Autodesk Inventor part; units mm, degrees
ref_plane "YZ Plane" through (0, 0, 0) normal (1, 0, 0) x (0, 1, 0)
ref_plane "XZ Plane" through (0, 0, 0) normal (0, 1, 0) x (-1, 0, 0)
ref_plane "XY Plane" through (0, 0, 0) normal (0, 0, 1) x (1, 0, 0)
sketch "Sketch1" plane through (0, 0, 0) normal (0, 0, 1) x (1, 0, 0)
  circle A0 centre (0, 0) radius 75 construction
  arc A1 (-78.5195, 32.5529) -> (0, 0) centre (-15.5934, 73.3611) ccw
  line L0 (-15.5934, 73.3611) -> (-78.5195, 32.5529) construction
  line L1 (-15.5934, 73.3611) -> (0, 0) construction
  line L2 (0, 0) -> (64.9519, 37.5) construction
  arc A2 (6.6958, 84.7359) -> (0, 0) centre (64.9519, 37.5) ccw
  line L3 (64.9519, 37.5) -> (6.6958, 84.7359) construction
  line L4 (64.9519, 37.5) -> (0, 0) construction
  line L5 (0, 0) -> (0, 75) construction
  circle A3 centre (0, 0) radius 85 construction
  arc A4 (6.6958, 84.7359) -> (-78.5195, 32.5529) centre (0, 0) ccw
  arc A5 (-74.153, 41.5492) -> (-78.5195, 32.5529) centre (-76.3362, 37.0511) ccw
  line L6 (-76.3362, 37.0511) -> (-78.5195, 32.5529) construction
  line L7 (-76.3362, 37.0511) -> (-74.153, 41.5492) construction
  point P0 (0, 0)
  dimension "d1" = 72
  dimension "d4" = 60
  dimension "d21" = 170
  dimension "d39" = 5
  dimension "d40" = 180
extrude "Extrusion1" add sketch "Sketch1" along normal blind 10
sketch "Sketch3" plane through (0, 0, 10) normal (0, 0, 1) x (1, 0, 0)
  circle A0 centre (0, 0) radius 80 construction
  circle A1 centre (64.9519, 37.5) radius 75
  circle A2 centre (64.9519, 37.5) radius 80 construction
  point P0 (0, 0)
  point P1 (-2.8573, 79.949)
  dimension "d25" = 160
  dimension "d26" = 160
hole "Hole2" at (-2.8573, 79.949, 10) direction (0, 0, -1) diameter 5 end through all
sketch "Sketch4" plane through (0, 0, 10) normal (0, 0, 1) x (1, 0, 0)
  circle A0 centre (-2.8573, 79.949) radius 2.5
  arc A1 (-78.5195, 32.5529) -> (0, 0) centre (-15.5934, 73.3611) ccw
  arc A2 (6.6958, 84.7359) -> (1.3808, 77.2959) centre (64.9519, 37.5) ccw
  arc A3 (6.6958, 84.7359) -> (-3.0359, 84.9458) centre (0, 0) ccw
  arc A4 (6.6958, 84.7359) -> (0, 0) centre (64.9519, 37.5) ccw
  arc A5 (6.6958, 84.7359) -> (-78.5195, 32.5529) centre (0, 0) ccw
  circle A6 centre (-2.8573, 79.949) radius 5
extrude "Extrusion2" cut sketch "Sketch4" against normal blind 10 contours A3 A2 A6
sketch "Sketch5" plane through (0, 0, 10) normal (0, 0, 1) x (1, 0, 0)
  arc A0 (1.3808, 77.2959) -> (-3.0359, 84.9458) centre (-2.8573, 79.949) ccw
  arc A1 (-3.0359, 84.9458) -> (-74.153, 41.5492) centre (0, 0) ccw
  arc A2 (-74.153, 41.5492) -> (-78.5195, 32.5529) centre (-76.3362, 37.0511) ccw
  arc A3 (-78.5195, 32.5529) -> (0, 0) centre (-15.5934, 73.3611) ccw
  arc A4 (1.3808, 77.2959) -> (0, 0) centre (64.9519, 37.5) ccw
  circle A5 centre (-2.8573, 79.949) radius 2.5
  point P0 (0, 0)
hole "Hole3" at (-76.3362, 37.0511, 10) direction (0, 0, -1) diameter 4.134 end through all
sketch "Sketch7" plane through (0, 0, 0) normal (0, 0, -1) x (-1, 0, 0)
  circle A0 centre (76.3362, 37.0511) radius 2.067
  arc A1 (3.0359, 84.9458) -> (-1.3808, 77.2959) centre (2.8573, 79.949) ccw
  arc A2 (0, 0) -> (-1.3808, 77.2959) centre (-64.9519, 37.5) ccw
  arc A3 (0, 0) -> (78.5195, 32.5529) centre (15.5934, 73.3611) ccw
  arc A4 (78.5195, 32.5529) -> (74.153, 41.5492) centre (76.3362, 37.0511) ccw
  arc A5 (74.153, 41.5492) -> (3.0359, 84.9458) centre (0, 0) ccw
  circle A6 centre (2.8573, 79.949) radius 2.5
  arc A7 (71.5064, 35.8724) -> (12.5647, 79.0071) centre (0, 0) ccw
  arc A8 (14.8454, 3.3651) -> (70.9945, 30.5742) centre (15.5934, 73.3611) ccw
  arc A9 (10.2017, 10.0786) -> (7.2658, 71.9181) centre (-64.9519, 37.5) ccw
  arc A10 (10.2017, 10.0786) -> (14.8454, 3.3651) centre (14.8988, 8.3648) ccw
  arc A11 (12.5647, 79.0071) -> (7.2658, 71.9181) centre (11.7794, 74.0692) ccw
  arc A12 (70.9945, 30.5742) -> (71.5064, 35.8724) centre (67.0373, 33.6304) ccw
  point P0 (0, 0)
  dimension "d51" = 5
  dimension "d55" = 5
extrude "Extrusion4" cut sketch "Sketch7" against normal blind 2 contours A12 A8 A10 A9 A11 A7
properties part number "blad"
Read the model definition and answer for the solid it produces. Units are mm, in the model's axes. A direction names the side the tool comes from. Give positions to 0.01 mm unless a question says otherwise; leave off trailing zeros. Write each loop counter-clockwise with the first axis right and the second up, starting at its lowest first coordinate (ties: lowest second). Pieces come first, ordered by that corner, then holes. Notation, with made-up numbers: M 23.5,5.25 L 81.5,5.25 A16 ccw 81.5,17.25 Z; hole C 22,-26 d5. An arc over 180 degrees is marked long. One line per item, written item: value. Start each with the question number.
(1) Find section C-C (y = 67.5). Determine the outline of the cut face in (x, z).
(2) Determine the mould class of faces 1 (the cylindrical face through (-43.73, 3.84, 4.93)), 2 (the cylindrical face through (-76.96, 35.08, 4.93)), 3 (the flat face through (-31, 42, 10)) for opening direction Y: pulls with the +Y half, pulls with the -Y half, needs draft (parallel to the pull), parting line crosses it, or undercut.
(3) Find the intervals of material crossed by line 1 (Z direction, x = -39.5, y = 67); line 2 (X direction, y = 78.5, z = 3); line 3 (X direction, y = 28, z = 1.75), in increasing order.
(4) Flat-ended cylindrical pins translate along their axes: pin 1 Ø2 at (y, z) = (24, 5.5) entering from +X; pin 2 Ø3.5 at (x, y) = (-76.34, 37.05) entering from +Z; pin 3 Ø6 at (y, z) = (62.5, 1.5) entering from +X; pin 4 Ø1.5 at (x, z) = (-28, 2) entering from +Y. Find the tip coordinate at first contact, or state that the pin passes through.
(5) Find section B-B (x = -18). Determine the outline of the cut face in (y, z), plus the area to 3 significant figures.
(6) Find section A-A (z = 7). Determine the outline of the cut face in (x, y), plus the area to 3 significant figures.
(7) A tool of negligible diameter and unlimited length cuts with its end or side. For faces 4 (the cylindrical face through (-48, 64, 1)), 5 (the cylindrical face through (-3.608, 77.564, 4.93)), from which of +Z, -Z, +X, -X, +Y, -Y can it reach the whole face along a straight path? Write none if from no direction.
Results below:
1. outline: M -51.66,0 L -42.94,0 L -42.94,2 L -9.21,2 L -9.21,0 L -3.79,0 L -3.79,10 L -51.66,10 Z
2. face 1: pulls with the -Y half
2. face 2: undercut
2. face 3: needs draft
3. line 1: z = 2 to 10
3. line 2: x = -32.6 to -4.89, -0.82 to 1.93
3. line 3: x = -75.32 to -68.91, -14.48 to -9.44
4. pin 1: stops at x = -8.63
4. pin 2: passes through
4. pin 3: stops at x = -4.63
4. pin 4: stops at y = 80.51
5. outline: M -1.6,0 L 3.4,0 L 3.4,2 L 77.95,2 L 77.95,0 L 83.07,0 L 83.07,10 L -1.6,10 Z
5. area: 698 mm^2
6. outline: M -78.52,32.55 A75 ccw 0,0 A75 cw 1.38,77.3 A5 ccw -3.04,84.95 A85 ccw -74.15,41.55 A5 ccw Z; hole C -76.34,37.05 d4.13; hole C -2.86,79.95 d5
6. area: 4,520 mm^2
7. face 4: -Z
7. face 5: +Z, -Z
